```python
from build123d import *

# Parameters (mm, degrees)
BOSS_EXTRUDE1_DEPTH                   = 6.35
F_23_0_154_DIAMETER_HOLE1_D           = 3.9116
F_23_0_154_DIAMETER_HOLE1_CSINK_D     = 5.1816
F_23_0_154_DIAMETER_HOLE1_CSINK_ANGLE = 90
LPATTERN1_COUNT                       = 4
LPATTERN1_PITCH                       = 7.9375
LPATTERN1_COUNT_DIR2                  = 3
LPATTERN1_PITCH_DIR2                  = 7.9375


with BuildPart() as part:
    # Sketch1 → Boss-Extrude1 (new body)
    with BuildSketch(Plane.XY):
        with BuildLine():
            Line((-25.4, 0), (0, 0))
            Line((0, 0), (0, 33.02))
            Line((0, 33.02), (-19.576328296, 33.02))
            Line((-19.576328296, 33.02), (-33.216892644, 13.539255216))
            Line((-33.216892644, 13.539255216), (-31.734093122, 10.970971108))
            ThreePointArc((-31.734093122, 10.970971108), (-28.382856233, 8.341458547), (-27.78125, 4.124445986))
            Line((-27.78125, 4.124445986), (-25.4, 0))
        make_face()
        with BuildLine():
            Line((-31.734093122, 10.970971108), (-33.216892644, 13.539255216))
            Line((-33.216892644, 13.539255216), (-35.037997829, 10.938447476))
            ThreePointArc((-35.037997829, 10.938447476), (-33.388447139, 11.198681663), (-31.734093122, 10.970971108))
        make_face()
    extrude(amount=BOSS_EXTRUDE1_DEPTH)

    # #23 (0.154) Diameter Hole1 (through all)
    with Locations(Plane(origin=(-4.7625, 4.7625, 6.35), x_dir=(1, 0, 0), z_dir=(0, 0, 1))):
        with Locations((0, 0)):
            f_23_0_154_diameter_hole1 = CounterSinkHole(F_23_0_154_DIAMETER_HOLE1_D / 2, F_23_0_154_DIAMETER_HOLE1_CSINK_D / 2, counter_sink_angle=F_23_0_154_DIAMETER_HOLE1_CSINK_ANGLE)

    # LPattern1: 23 _0.154_ Diameter Hole1 4 × 3, 1 skipped
    with Locations(*[(-j * LPATTERN1_PITCH_DIR2, i * LPATTERN1_PITCH, 0) for i in range(LPATTERN1_COUNT) for j in range(LPATTERN1_COUNT_DIR2) if (i, j) not in ((0, 0), (3, 2))]):
        add(f_23_0_154_diameter_hole1, mode=Mode.SUBTRACT)


solid = part.part
```
Source: CAD feature listing. Evaluate the final solid. Frame: model axes, mm. Give positions to 0.01 mm unless a question says otherwise; leave off trailing zeros. Loops run counter-clockwise (first coordinate to the right, second up) from the corner with the lowest first, then second, coordinate; pieces in that order, holes last. Notation, with made-up numbers: (17.25, -23.75) - (57.25, -23.75) arc R10 cw to (57.25, -10.75) - close; hole circle Ø8 at (0, 18.25). An arc over 180 degrees is marked (long way). Use CSV: the item, a comma, the result in double quotes.
1) Mould query, pull axis Y, two halves, no side actions, for faces 1 (the cylindrical face through (-5.665, 10.965, 2.817)), 2 (the flat face through (-14, 17, 0)), 3 (the flat face through (-10, 33.02, 3)). Classes: +Y half, -Y half, draft (parallel to the pull), parting line (faces both ways), or undercut.
Worked out:
face 1,"undercut"
face 2,"draft"
face 3,"+Y half"
2) Cut plane D-D (x = -29.5). Output: boundary loops of the cut face in (y, z).
Worked out:
outline,"(9.72, 0) - (18.85, 0) - (18.85, 6.35) - (9.72, 6.35) - close"
3) Cut plane A-A (x = -12.7). Output: boundary loops of the cut face in (y, z) (3 decimals).
Worked out:
outline,"(0, 0) - (2.807, 0) - (2.807, 5.715) - (2.172, 6.35) - (0, 6.35) - close; (6.718, 0) - (10.744, 0) - (10.744, 5.715) - (10.109, 6.35) - (7.353, 6.35) - (6.718, 5.715) - close; (14.656, 0) - (18.682, 0) - (18.682, 5.715) - (18.047, 6.35) - (15.291, 6.35) - (14.656, 5.715) - close; (22.593, 0) - (26.619, 0) - (26.619, 5.715) - (25.984, 6.35) - (23.228, 6.35) - (22.593, 5.715) - close; (30.531, 0) - (33.02, 0) - (33.02, 6.35) - (31.166, 6.35) - (30.531, 5.715) - close"
4) Pin query (flat end, axial travel): P1, Ø6.5, axis at x = -20.64, y = 20.64, coming from the -Z side. Return the tip coordinate at first contact, or that it passes through.
Worked out:
P1,"stops at z = 0"
5) Cut plane B-B (y = 12.7). Output: boundary loops of the cut face in (x, z) (3 decimals), and give its area (3 significant figures).
Worked out:
outline,"(-33.805, 0) - (-22.593, 0) - (-22.593, 5.715) - (-23.228, 6.35) - (-33.805, 6.35) - close; (-18.682, 0) - (-14.656, 0) - (-14.656, 5.715) - (-15.291, 6.35) - (-18.047, 6.35) - (-18.682, 5.715) - close; (-10.744, 0) - (-6.718, 0) - (-6.718, 5.715) - (-7.353, 6.35) - (-10.109, 6.35) - (-10.744, 5.715) - close; (-2.807, 0) - (0, 0) - (0, 6.35) - (-2.172, 6.35) - (-2.807, 5.715) - close"
area,"139 mm^2"
6) Cut plane C-C (z = 4.25). Count the separate pieces of the cut face and the enclosed holes in it, and give its area (3 significant figures).
Worked out:
separate pieces,"1"
enclosed holes,"11"
area,"774 mm^2"
7) Line query: line 1 (Y direction, x = -12.7, z = 3.7); line 2 (X direction, y = 13.5, z = 3); line 3 (X direction, y = 14, z = 2.25). Output: solid intervals per line, ascending.
Worked out:
line 1,"y = 0 to 2.81, 6.72 to 10.74, 14.66 to 18.68, 22.59 to 26.62, 30.53 to 33.02"
line 2,"x = -33.24 to -22.42, -18.85 to -14.48, -10.92 to -6.55, -2.98 to 0"
line 3,"x = -32.89 to -22.1, -19.18 to -14.16, -11.24 to -6.22, -3.3 to 0"
